Here's how the part is built. I have some questions about the finished solid (model axes, mm). Face numbers are marked on the shaded views. Give positions to 0.01 mm unless a question says otherwise; leave off trailing zeros. Write each loop counter-clockwise with the first axis right and the second up, starting at its lowest first coordinate (ties: lowest second). Pieces come first, ordered by that corner, then holes. Notation, with made-up numbers: (72, -24) -> (130, -24) arc R15 ccw to (130, -17) -> close; hole circle Ø8 at (14, 44.5). An arc over 180 degrees is marked (long way). Return JSON: item names as keys, results as strings.
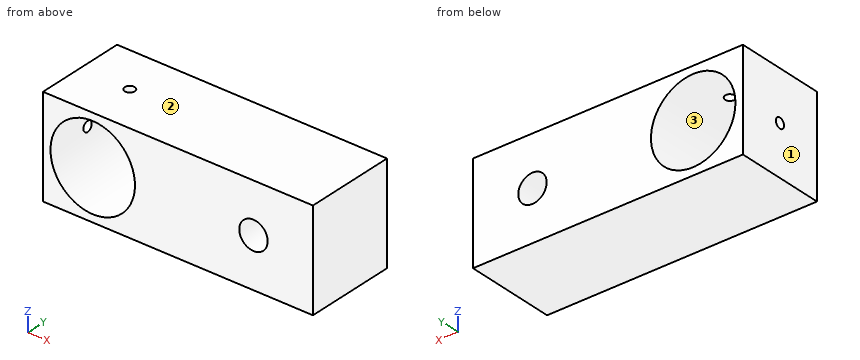
Autodesk Inventor part; units mm, degrees
ref_plane "YZ Plane" through (0, 0, 0) normal (1, 0, 0) x (0, 1, 0)
ref_plane "XZ Plane" through (0, 0, 0) normal (0, 1, 0) x (-1, 0, 0)
ref_plane "XY Plane" through (0, 0, 0) normal (0, 0, 1) x (1, 0, 0)
sketch "Sketch1" plane through (0, 0, 0) normal (0, 1, 0) x (-1, 0, 0)
  circle A0 centre (0, 0) radius 14.875
  line L0 (-17.5, 17.5) -> (17.5, 17.5)
  line L1 (17.5, 17.5) -> (17.5, -17.5)
  line L2 (17.5, -17.5) -> (-17.5, -17.5)
  line L3 (-17.5, -17.5) -> (-17.5, 17.5)
  line L4 (-17.5, 17.5) -> (17.5, -17.5) construction
  line L5 (17.5, 17.5) -> (-17.5, -17.5) construction
  dimension "d0" = 29.75
  dimension "d1" = 35
  dimension "d2" = 35
extrude "Extrusion1" add sketch "Sketch1" along normal blind 32
sketch "Sketch2" plane through (17.5, 0, 17.5) normal (1, 0, 0) x (0, 0, -1)
  line L0 (0, 0) -> (35, 0)
  line L1 (35, 0) -> (35, 32)
  line L2 (35, 32) -> (0, 32)
  line L3 (0, 32) -> (0, 0)
  point P0 (17.5, 0)
sketch "Sketch3" plane through (0, 32, 0) normal (0, 1, 0) x (1, 0, 0)
  line L0 (17.5, -17.5) -> (17.5, 17.5)
  line L1 (17.5, 0) -> (56.57, 0)
  circle A0 centre (56.57, 0) radius 5
  point P0 (0, 0)
  dimension "d5" = 56.57
  dimension "d9" = 10
extrude "Extrusion2" add sketch "Sketch2" along normal blind 60
extrude "Extrusion3" cut sketch "Sketch3" against normal through all
sketch "Sketch5" plane through (-17.5, 0, 17.5) normal (0, 0, 1) x (1, 0, 0)
  circle A0 centre (17.5, 16) radius 1.778
  point P0 (17.5, 0)
  dimension "d15" = 3.556
extrude "Extrusion5" cut sketch "Sketch5" against normal blind 10
sketch "Sketch6" plane through (-17.5, 0, -17.5) normal (-1, 0, 0) x (0, 0, 1)
  circle A0 centre (17.5, 16) radius 1.778
  point P0 (17.5, 0)
  dimension "d18" = 3.556
extrude "Extrusion6" cut sketch "Sketch6" against normal blind 3.556
equation "\"d19\" = d18"
properties part number "MotorBarConnect"
1. Suppose I cut it at B-B, the plane x = 0. List the corners of the cut face in (y, z) for me (3 decimals).
Taken from the geometry:
{"outline": "(0, -17.5) -> (32, -17.5) -> (32, -14.875) -> (0, -14.875) -> close; (0, 14.875) -> (14.222, 14.875) -> (14.222, 17.5) -> (0, 17.5) -> close; (17.778, 14.875) -> (32, 14.875) -> (32, 17.5) -> (17.778, 17.5) -> close"}
2. Suppose I cut it at C-C, the plane z = 12.5. List the corners of the cut face in (x, y) for me.
Taken from the geometry:
{"outline": "(-17.5, 0) -> (-8.06, 0) -> (-8.06, 32) -> (-17.5, 32) -> close; (8.06, 0) -> (77.5, 0) -> (77.5, 32) -> (8.06, 32) -> close"}
3. Suppose I cut it at D-D, the plane x = 56.57. List the corners of the cut face in (y, z) for me.
Taken from the geometry:
{"outline": "(0, -17.5) -> (32, -17.5) -> (32, -5) -> (0, -5) -> close; (0, 5) -> (32, 5) -> (32, 17.5) -> (0, 17.5) -> close"}
4. If we mould it in two halves opening along Z, with no side actions, what happens to the marked faces 1, 2 and 3? For each: released by +Z, released by -Z, zero draft, split by the parting line, or undercut.
Taken from the geometry:
{"face 1": "zero draft", "face 2": "released by +Z", "face 3": "undercut"}
5. If I drill on line 1 (X direction, y = 5, z = -2.5); line 2 (X direction, y = 16, z = 15.65); line 3 (Z direction, x = -15.95, y = 16), over which ranges is the centre line in solid material (lowest first)? Write a range as [from, to].
Taken from the geometry:
{"line 1": "x = [-17.5, -14.66], [14.66, 52.24], [60.9, 77.5]", "line 2": "x = [-17.5, -1.78], [1.78, 77.5]", "line 3": "z = [-17.5, -1.78], [1.78, 17.5]"}
6. Suppose I cut it at A-A, the plane y = 16. List the corners of the cut face in (x, z) for me (3 decimals).
Taken from the geometry:
{"outline": "(-17.5, -17.5) -> (77.5, -17.5) -> (77.5, 17.5) -> (1.778, 17.5) -> (1.778, 14.768) arc R14.875 cw (long way) to (-14.768, -1.778) -> (-17.5, -1.778) -> close; (-17.5, 1.778) -> (-14.768, 1.778) arc R14.875 cw to (-1.778, 14.768) -> (-1.778, 17.5) -> (-17.5, 17.5) -> close; hole circle Ø10 at (56.57, 0)"}
